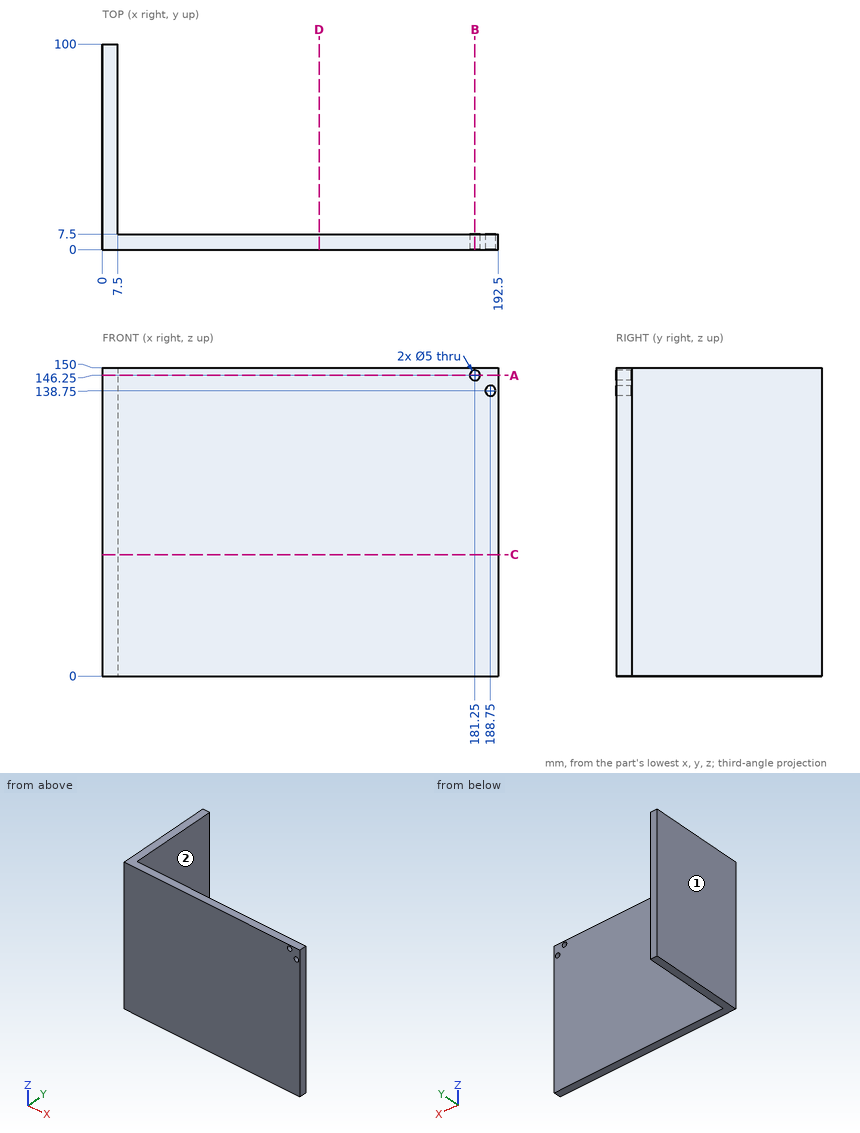
Can you work these out from the drawing? Everything is in mm from the part's minimum corner. A direction names the side the tool comes from. Give positions to 0.01 mm unless a question says otherwise; leave off trailing zeros. Loops run counter-clockwise (first coordinate to the right, second up) from the corner with the lowest first, then second, coordinate; pieces in that order, holes last. Notation, with made-up numbers: (-19.75, -5) -> (18.25, -5) arc R9 ccw to (18.25, 4) -> close; hole circle Ø7 at (77.25, 12.5). An arc over 180 degrees is marked (long way). Write item = value, one per line.
1) For the marked faces 1 and 2, which set-ups out of +Z, -Z, +X, -X, +Y, -Y let a thin tool reach every point of the face, with its end or its side?
Check result:
face_1 = +Z, -Z, -X, +Y, -Y
face_2 = +Z, -Z, +X, +Y
2) Suppose I cut it at C-C on z = 59. Write out the boundary of the cut face in (x, y).
Check result:
outline = (0, 0) -> (192.5, 0) -> (192.5, 7.5) -> (7.5, 7.5) -> (7.5, 100) -> (0, 100) -> close
3) Suppose I cut it at A-A on z = 146.25. Write out the boundary of the cut face in (x, y), then the cut area to 3 significant figures.
Check result:
outline = (0, 0) -> (178.75, 0) -> (178.75, 7.5) -> (7.5, 7.5) -> (7.5, 100) -> (0, 100) -> close; (183.75, 0) -> (192.5, 0) -> (192.5, 7.5) -> (183.75, 7.5) -> close
area = 2,100 mm2
4) Suppose I cut it at D-D on x = 105.5. Write out the boundary of the cut face in (y, z).
Check result:
outline = (0, 0) -> (7.5, 0) -> (7.5, 150) -> (0, 150) -> close
5) Suppose I cut it at B-B on x = 181.25. Write out the boundary of the cut face in (y, z).
Check result:
outline = (0, 0) -> (7.5, 0) -> (7.5, 143.75) -> (0, 143.75) -> close; (0, 148.75) -> (7.5, 148.75) -> (7.5, 150) -> (0, 150) -> close
6) Will these pins go through, and if not, where does the flat tip stop? pin 1 (1.5 mm diameter, centred on y = 24.5, z = 17.5, fed in from +X); pin 2 (6.5 mm diameter, centred on x = 188.75, z = 138.75, fed in from +Y).
Check result:
pin_1 = 7.5
pin_2 = 7.5
7) I need wall thicknesses on L1, parallel to X at y = 4, z = 146.25; L2, parallel to X at y = 5, z = 138.75; L3, parallel to Z at x = 188.75, y = 4.75. Which ranges of each line are inside material? Lowest first, please. Write a range as from..to.
Check result:
L1 = 0..178.75, 183.75..192.5
L2 = 0..186.25, 191.25..192.5
L3 = 0..136.25, 141.25..150
